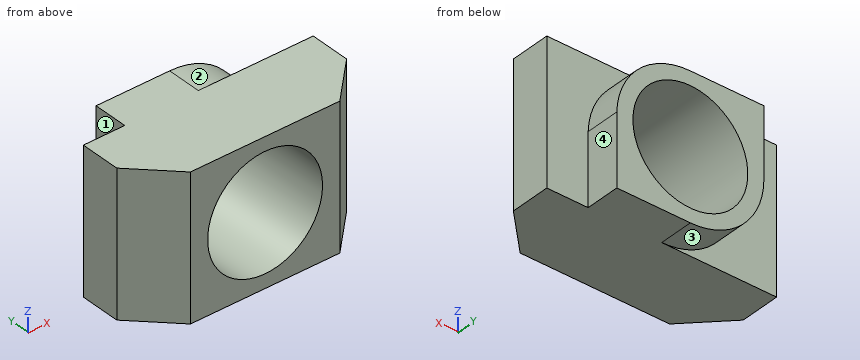
```python
from build123d import *

# Parameters (mm, degrees)
BOSS_EXTRUDE1_DEPTH = 6.2
SKETCH2_R           = 2.5
CUT_EXTRUDE1_DEPTH  = 8
CUT_EXTRUDE2_DEPTH  = 1.5


with BuildPart() as part:
    # Sketch1 → Boss-Extrude1 (new body)
    with BuildSketch(Plane.XY):
        Polygon((0, 5), (0, 0), (3.25, 0), (5, 1.75), (5, 3.5), (3.2, 3.5), (3.2, 5), align=None)
    extrude(amount=BOSS_EXTRUDE1_DEPTH)

    # Mirror1: part across plane


with BuildPart() as part_1:
    add(part.part)
    add(part.part.mirror(Plane(origin=(0, 0, 0), x_dir=(0, 0, 1), z_dir=(1, 0, 0))))

    # Sketch2 → Cut-Extrude1 (cut)
    with BuildSketch(Plane(origin=(0, 5, 0), x_dir=(1, 0, 0), z_dir=(0, 1, 0))):
        with Locations((0, -3.1)):
            Circle(SKETCH2_R)
    extrude(amount=-CUT_EXTRUDE1_DEPTH, mode=Mode.SUBTRACT)

    # Sketch3 → Cut-Extrude2 (cut)
    with BuildSketch(Plane(origin=(0, 5, 0), x_dir=(1, 0, 0), z_dir=(0, 1, 0))):
        with BuildLine():
            ThreePointArc((3.2, -3.1), (2.227666941, -5.297914262), (0, -6.2))
            Line((0, -6.2), (3.2, -6.2))
            Line((3.2, -6.2), (3.2, -3.1))
        make_face()
        with BuildLine():
            Line((-3.2, 0), (-3.2, -3.2))
            ThreePointArc((-3.2, -3.2), (-2.2627417, -0.9372583), (0, 0))
            Line((0, 0), (-3.2, 0))
        make_face()
    extrude(amount=-CUT_EXTRUDE2_DEPTH, mode=Mode.SUBTRACT)


solid = part_1.part
```
Here's how the part is built. I have some questions about the finished solid (model axes, mm). Face numbers are marked on the shaded views. A direction names the side the tool comes from. Round coordinates to 2 decimals unless told otherwise and drop trailing zeros. Loops run counter-clockwise (first coordinate to the right, second up) from the corner with the lowest first, then second, coordinate; pieces in that order, holes last.
1. Suppose I cut it at C-C, the plane x = -0.75. Please give me the cut outline in (y, z).
Answers:
outline: (0, 0) - (3.5, 0) - (3.5, 0.09) - (5, 0.09) - (5, 0.72) - (0, 0.72) - close; (0, 5.48) - (5, 5.48) - (5, 6.2) - (0, 6.2) - close
2. Suppose I cut it at B-B, the plane z = 2. Please give me the cut outline in (x, y) (3 decimals).
Answers:
outline: (-5, 1.75) - (-3.25, 0) - (-2.245, 0) - (-2.245, 5) - (-2.966, 5) - (-2.966, 3.5) - (-5, 3.5) - close; (2.245, 0) - (3.25, 0) - (5, 1.75) - (5, 3.5) - (3.2, 3.5) - (3.2, 5) - (2.245, 5) - close
3. Will these pins go through, and if not, where does the flat tip stop? pin 1 (2 mm diameter, centred on x = -3.5, z = 2, fed in from -Y); pin 2 (1.2 mm diameter, centred on y = 4.5, z = 1.5, fed in from +X); pin 3 (1.5 mm diameter, centred on x = -4, z = 3.5, fed in from +Y); pin 4 (1.6 mm diameter, centred on y = 4.5, z = 4, fed in from -X).
Answers:
pin 1: stops at y = 0
pin 2: stops at x = 3.2
pin 3: stops at y = 3.5
pin 4: stops at x = -3.2
4. If I drill on probe 1 along Z at (x, y) = (0, 2.5); probe 2 along X at (y, z) = (3.6, 3.1); probe 3 along X at (y, z) = (2, 3.1), over which ranges is the centre line in solid material (lowest first)?
Answers:
probe 1: z = 0 to 0.6, 5.6 to 6.2
probe 2: x = -3.2 to -2.5, 2.5 to 3.2
probe 3: x = -5 to -2.5, 2.5 to 5
5. Suppose I cut it at D-D, the plane y = 2.9. Please give me the cut outline in (x, z), and give its area (3 significant figures).
Answers:
outline: (-5, 0) - (5, 0) - (5, 6.2) - (-5, 6.2) - close; hole circle Ø5 at (0, 3.1)
area: 42.4 mm2
6. For the marked faces 1, 2, 3 and 4, which set-ups out of +Z, -Z, +X, -X, +Y, -Y let a thin tool reach every point of the face, with its end or its side?
Answers:
face 1: +Z, -Z, -X, +Y
face 2: +Z, +X, +Y
face 3: -Z, -X, +Y
face 4: +Z, -Z, +X, +Y
7. Suppose I cut it at A-A, the plane y = 0.8. Please give me the cut outline in (x, z).
Answers:
outline: (-4.05, 0) - (4.05, 0) - (4.05, 6.2) - (-4.05, 6.2) - close; hole circle Ø5 at (0, 3.1)
